Verification items for the finished model (mm, model axes). A direction names the side the tool comes from. Give positions to 0.01 mm unless a question says otherwise; leave off trailing zeros. Write each loop counter-clockwise with the first axis right and the second up, starting at its lowest first coordinate (ties: lowest second). Pieces come first, ordered by that corner, then holes. Notation, with made-up numbers: (73.5, 87.5) -> (108.5, 87.5) arc R22 ccw to (108.5, 116.5) -> close; hole circle Ø8 at (24, -16). An arc over 180 degrees is marked (long way). Use one line per item in the form item = value. Start each with the question number.
(1) Scan lines: L1, parallel to Z at x = 4.5, y = 0; L2, parallel to Y at x = 1.75, z = -0.25; L3, parallel to X at y = -5.5, z = -1.75. Record each from-to range of solid material in increasing order.
(2) Set-up check for faces 1 (the face through (4.653, 4.31, -2.535)), 2 (the face through (2.501, -4.6, 2.7)), 3 (the face through (5, 0, -5)): record each of +Z, -Z, +X, -X, +Y, -Y from which the full face is reachable in a straight line by a thin tool's end or side.
(3) Release check for a two-part mould opening along Z. For faces 4 (the face through (4.653, -4.31, 2.535)), 5 (the face through (3.855, -0.738, 2.345)), 6 (the face through (0, -3, -1)) record: pulls with the +Z half, pulls with the -Z half, needs draft (parallel to the pull), parting line crosses it, or undercut.
(4) Depth check by flat-ended pin: pin 1 Ø1 at (y, z) = (-4.5, -5.5) entering from -X; pin 2 Ø0.9 at (y, z) = (-4.5, -2) entering from +X; pin 3 Ø4 at (x, y) = (2, 2) entering from -Z. Enter the tip coordinate at first touch or a pass-through.
(5) Section check B-B, the plane x = 2.25. Record the cut outline in (y, z), plus the area to 3 significant figures.
(6) Section check A-A, the plane y = 0. Record the cut outline in (x, z).
Autodesk Inventor part; units mm, degrees
ref_plane "Work Plane1" through (21.3675, 0, 0) normal (0, 0, -1) x (-1, 0, 0)
ref_plane "YZ Plane" through (0, 0, 0) normal (1, 0, 0) x (0, 1, 0)
ref_plane "XZ Plane" through (0, 0, 0) normal (0, 1, 0) x (-1, 0, 0)
sketch "Esquisse1" plane through (0, 0, 0) normal (0, 0, 1) x (1, 0, 0)
  line L0 (-1.7132, 0) -> (8.8022, 0)
  line L1 (2.5009, 5.7735) -> (2.0526, 6.55)
  line L2 (2.5009, 5.7735) -> (7.3, 5.7735) construction
  line L3 (7.3, 5.7735) -> (7.3, 0) construction
  arc A0 (2.0526, 6.55) -> (0, 6) centre (1.1, 6) ccw
  line L4 (2.5009, 5.7735) -> (2.5009, 0)
  line L5 (0, -1.4675) -> (0, 8.805)
  point P0 (0, 0)
  dimension "d2" = 11.547
  dimension "d4" = 14.2
  dimension "d5" = 1.1
  dimension "d15" = 7.3
  dimension "d16" = 30
revolve "Anneau" add sketch "Esquisse1" angle 360 about axis through (-10, 0, 0) along (1, 0, 0)
sketch "Esquisse2" plane through (0, 0, 0) normal (-1, 0, 0) x (0, 0, 1)
  circle A0 centre (0, 0) radius 4.9
  line L0 (-5, -2.8868) -> (-5, 2.8868)
  line L1 (-5, 2.8868) -> (0, 5.7735)
  line L2 (0, 5.7735) -> (5, 2.8868)
  line L3 (5, 2.8868) -> (5, -2.8868)
  line L4 (5, -2.8868) -> (0, -5.7735)
  line L5 (0, -5.7735) -> (-5, -2.8868)
  circle A1 centre (0, 0) radius 6
  dimension "d6" = 11.547
extrude "Corps" add sketch "Esquisse2" against normal blind 7.3 contours A0 | L0 L1 L2 L3 L4 L5
sketch "Esquisse3" plane through (0, 0, 0) normal (0, 0, 1) x (1, 0, 0)
  line L0 (2.5009, 5.7735) -> (7.3, 5.7735)
  line L1 (7.3, 2.8868) -> (7.3, 5.7735)
  line L2 (0, -6) -> (0, 6)
  line L3 (-1.46, 0) -> (8.76, 0)
  line L4 (6.4204, 5.7735) -> (7.3, 4.25)
  dimension "d10" = 30
  dimension "d11" = 8.5
revolve "Chanfrein1" cut sketch "Esquisse3" angle 360 about axis through (-10, 0, 0) along (1, 0, 0)
sketch "Esquisse4" plane through (0, 0, 0) normal (-1, 0, 0) x (0, 0, 1)
  line L0 (-9.94, 0) -> (9.94, 0)
  line L1 (0, 9.94) -> (0, -9.94)
  point P0 (0, 0)
hole "Filetage" at (0, 0, 0) direction (1, 0, 0) diameter 4.917 end through all
chamfer "Chanfrein2" distance 0.5413 angle 30 1 edges at (0, 0, -2.4585) measured on face at (0, 4.7554, -0.5774)
ref_plane "Work Plane1" through (21.3675, 0, 0) normal (0, 0, -1) x (-1, 0, 0)
equation "\"d2\" = 1.1547 * SW"
equation "\"d4\" = LADI"
equation "\"d5\" = PHH"
equation "\"d15\" = KOH"
equation "\"d16\" = KEWI"
equation "\"d6\" = 1.1547 * SW"
equation "\"d7\" = KOH"
equation "\"d10\" = ANG1"
equation "\"d11\" = SW0"
equation "\"d12\" = -0.5 * GD1 + 0.5 * NND"
equation "\"d42\" = -0.5 * GD1 + 0.5 * NND"
equation "\"ANG1\" = 30deg"
equation "\"KEWI\" = 30deg"
equation "\"NND\" = 6"
equation "\"LADI\" = 14.2"
equation "\"PHH\" = 1.1"
equation "\"KOH\" = 7.3"
equation "\"SW0\" = 0.85 * SW"
equation "\"d1\" = LADI"
equation "\"d3\" = PHH"
equation "\"GUL\" = 0.541266 * PTC"
equation "\"THREADDIA\" = 6"
equation "\"TOA\" = 30deg"
equation "\"PTC\" = 1"
equation "\"GAL\" = 0.541266 * PTC"
equation "\"E0\" = 1.155 * SW"
properties part number "ANSI B18.16.3M - M6 x 1 Type de métal" material "Acier, doux"
Completed:
q1.L1 = -5 to -2.46, 2.46 to 5
q1.L2 = -6.88 to -2.45, 2.45 to 6.88
q1.L3 = 0 to 2.5
q2.face_1 = -Z, +X, +Y
q2.face_2 = +Z, +X, -Y
q2.face_3 = -Z, +X, +Y, -Y
q3.face_4 = pulls with the +Z half
q3.face_5 = undercut
q3.face_6 = needs draft
q4.pin_1 = 0.18
q4.pin_2 = 7.17
q4.pin_3 = -7.1
q5.outline = circle Ø12.42 at (0, 0); hole circle Ø4.92 at (0, 0)
q5.area = 102 mm²
q6.outline = (0, -6) arc R1.1 ccw to (2.05, -6.55) -> (2.5, -5.77) -> (2.5, -5) -> (6.87, -5) -> (7.3, -4.25) -> (7.3, -2.46) -> (0.31, -2.46) -> (0, -3) -> close; (0, 3) -> (0.31, 2.46) -> (7.3, 2.46) -> (7.3, 4.25) -> (6.87, 5) -> (2.5, 5) -> (2.5, 5.77) -> (2.05, 6.55) arc R1.1 ccw to (0, 6) -> close
